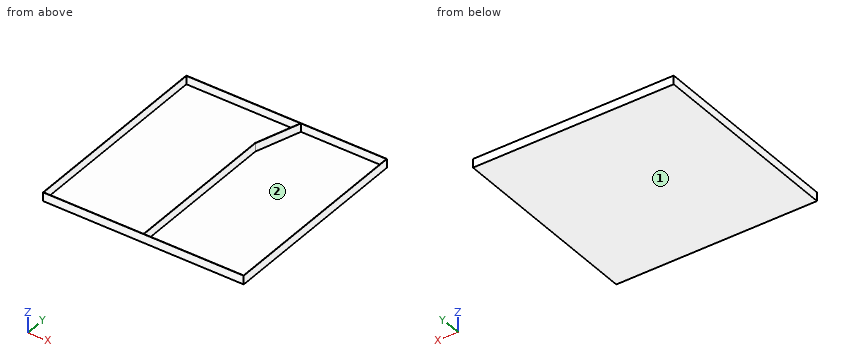
```python
from build123d import *

# Parameters (mm, degrees)
F0_W     = 600
F0_H     = 600
F1_DEPTH = 1
F2_W     = 600
F2_H     = 600
F3_DEPTH = 25


with BuildPart() as f1:
    # F0 (on Top) → F1 (new body)
    with BuildSketch(Plane.XY):
        Rectangle(F0_W, F0_H)
    extrude(amount=F1_DEPTH)

    # F2 (on face) → F3 (join)
    with BuildSketch(Plane.XY.offset(1)):
        Rectangle(F2_W, F2_H)
        Polygon((-299, -299), (-299, 299), (42.380814, 299), (0, 167.511806), (0, -299), align=None, mode=Mode.SUBTRACT)
        Polygon((43.431474, 299), (299, 299), (299, -299), (1, -299), (1, 167.354629), align=None, mode=Mode.SUBTRACT)
    extrude(amount=F3_DEPTH)


solid = f1.part
```
Here's how the part is built. I have some questions about the finished solid (model axes, mm). Face numbers are marked on the shaded views. Give positions to 0.01 mm unless a question says otherwise; leave off trailing zeros. Write each loop counter-clockwise with the first axis right and the second up, starting at its lowest first coordinate (ties: lowest second). Pieces come first, ordered by that corner, then holes. Notation, with made-up numbers: (-36.75, -6.75) -> (-8.75, -6.75) arc R10 ccw to (-8.75, 8.25) -> close; hole circle Ø4 at (62, -19.75). An arc over 180 degrees is marked (long way). Write each question's results on one line, items separated by ' | '.
Item 1: Suppose I cut it at C-C on x = -140. Write out the boundary of the cut face in (y, z).
Output:
outline: (-300, 0) -> (300, 0) -> (300, 26) -> (299, 26) -> (299, 1) -> (-299, 1) -> (-299, 26) -> (-300, 26) -> close
Item 2: Suppose I cut it at A-A on z = 17. Write out the boundary of the cut face in (x, y), plus the area to 3 significant figures.
Output:
outline: (-300, -300) -> (300, -300) -> (300, 300) -> (-300, 300) -> close; hole (-299, -299) -> (0, -299) -> (0, 167.51) -> (42.38, 299) -> (-299, 299) -> close; hole (1, -299) -> (299, -299) -> (299, 299) -> (43.43, 299) -> (1, 167.35) -> close | area: 3,000 mm^2
Item 3: We'd pull the mould along Y, two halves only. Please class the marked faces 1 and 2: pulls with the +Y half, pulls with the -Y half, needs draft (parallel to the pull), parting line crosses it, or undercut.
Output:
face 1: needs draft | face 2: undercut
Item 4: If I drill on L1, parallel to X at y = 14.5, z = 3.5; L2, parallel to Y at x = 223, z = 15.75; L3, parallel to Z at x = -185.5, y = 193, over which ranges is the centre line in solid material (lowest first)?
Output:
L1: x = -300 to -299, 0 to 1, 299 to 300 | L2: y = -300 to -299, 299 to 300 | L3: z = 0 to 1
Item 5: Suppose I cut it at B-B on y = -250. Write out the boundary of the cut face in (x, z), plus the area to 3 significant figures.
Output:
outline: (-300, 0) -> (300, 0) -> (300, 26) -> (299, 26) -> (299, 1) -> (1, 1) -> (1, 26) -> (0, 26) -> (0, 1) -> (-299, 1) -> (-299, 26) -> (-300, 26) -> close | area: 675 mm^2
Item 6: Suppose I cut it at D-D on y = 223. Write out the boundary of the cut face in (x, z), plus the area to 3 significant figures.
Output:
outline: (-300, 0) -> (300, 0) -> (300, 26) -> (299, 26) -> (299, 1) -> (18.94, 1) -> (18.94, 26) -> (17.88, 26) -> (17.88, 1) -> (-299, 1) -> (-299, 26) -> (-300, 26) -> close | area: 676 mm^2
Item 7: For pin 1 Ø12 at (x, y) = (119, 42.5) entering from -Z; pin 2 Ø12 at (x, y) = (-64, 66) entering from +Z, each with a flat end and sliding along its axis, tell me the tip position at first contact or that it passes through.
Output:
pin 1: stops at z = 0 | pin 2: stops at z = 1
